Study the drawing (mm; zero at the part's minimum x, y, z) and answer. A direction names the side the tool comes from. Coordinates: 2 decimals unless noted, no trailing zeros. Loops run counter-clockwise (first coordinate to the right, second up) from the corner with the lowest first, then second, coordinate; pieces in that order, holes last.
Q1. The mould has two halves that part along Z. Classify the marked faces 1, 2, 3 and 4: pulls with the +Z half, pulls with the -Z half, needs draft (parallel to the pull), parting line crosses it, or undercut.
Q2. Section A-A (y = 9) is taken. Give the vertices of the cut face in (x, z), then the cut area to 3 significant figures.
Q3. Section D-D (x = 19.5) is taken. Give the vertices of the cut face in (y, z).
Q4. Which of the six approach directions +Z, -Z, +X, -X, +Y, -Y give full straight-line access (tool end or side, diameter ignored) to the marked faces 5, 6 and 7?
Q5. Section C-C (z = 8.75) is taken. Give the vertices of the cut face in (x, y).
Q6. Section B-B (z = 4.5) is taken. Give the vertices of the cut face in (x, y).
Q7. Straight lines are drawn through the part: line 1 (X direction, y = 8, z = 2.5); line 2 (Z direction, x = 25, y = 7); line 3 (X direction, y = 6.75, z = 4.25). For each, find the intervals that lie inside material, in ascending order.
Q8. Flat-ended cylindrical pins translate along their axes: P1, Ø2.5, axis at x = 25.5, z = 6, coming from the -Y side; P2, Ø1.8, axis at x = 25, z = 5, coming from the -Y side; P3, Ø1, axis at y = 4, z = 7, coming from the +X side. Find the tip coordinate at first contact, or state that the pin passes through.
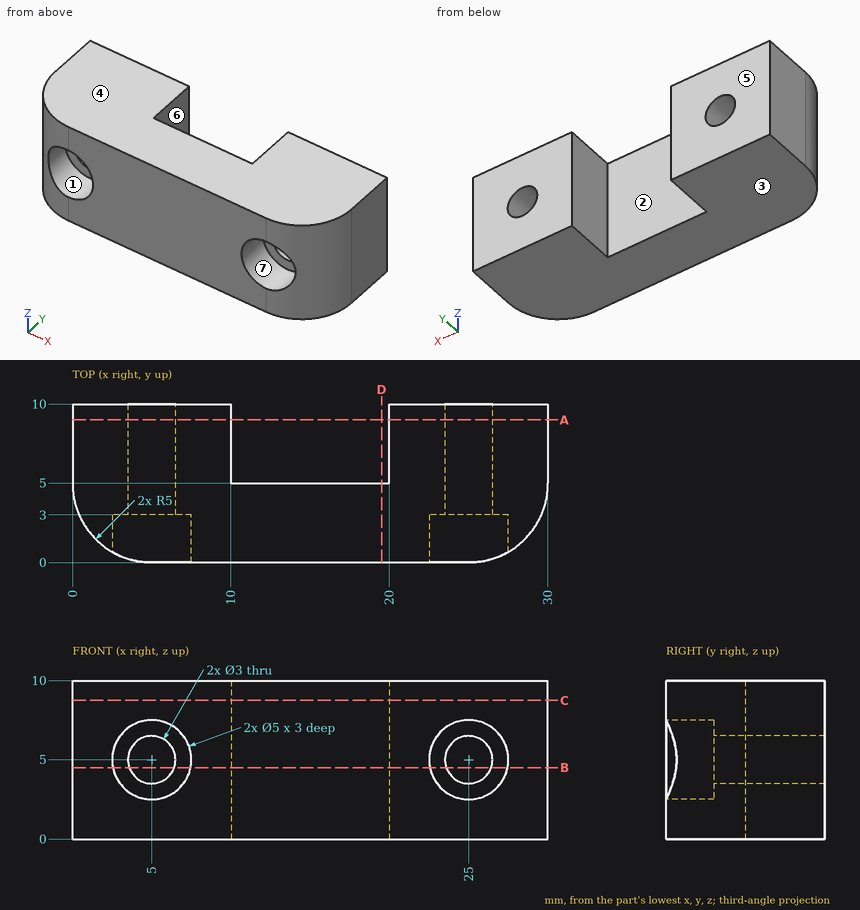
Numbers:
1. face 1: undercut
1. face 2: needs draft
1. face 3: pulls with the -Z half
1. face 4: pulls with the +Z half
2. outline: (0, 0) - (10, 0) - (10, 10) - (0, 10) - close; (20, 0) - (30, 0) - (30, 10) - (20, 10) - close; hole circle Ø3 at (5, 5); hole circle Ø3 at (25, 5)
2. area: 186 mm2
3. outline: (0, 0) - (5, 0) - (5, 10) - (0, 10) - close
4. face 5: +Z, -Z, +X, -X, +Y
4. face 6: +Z, -Z, +Y
4. face 7: -Y
5. outline: (0, 5) arc R5 ccw to (5, 0) - (25, 0) arc R5 ccw to (30, 5) - (30, 10) - (20, 10) - (20, 5) - (10, 5) - (10, 10) - (0, 10) - close
6. outline: (0, 5) arc R5 ccw to (2.55, 0.64) - (2.55, 3) - (3.59, 3) - (3.59, 10) - (0, 10) - close; (6.41, 3) - (7.45, 3) - (7.45, 0) - (22.55, 0) - (22.55, 3) - (23.59, 3) - (23.59, 10) - (20, 10) - (20, 5) - (10, 5) - (10, 10) - (6.41, 10) - close; (26.41, 3) - (27.45, 3) - (27.45, 0.64) arc R5 ccw to (30, 5) - (30, 10) - (26.41, 10) - close
7. line 1: x = 0 to 10, 20 to 30
7. line 2: z = 0 to 3.5, 6.5 to 10
7. line 3: x = 0 to 3.7, 6.3 to 10, 20 to 23.7, 26.3 to 30
8. P1: stops at y = 3
8. P2: passes through
8. P3: stops at x = 29.97
